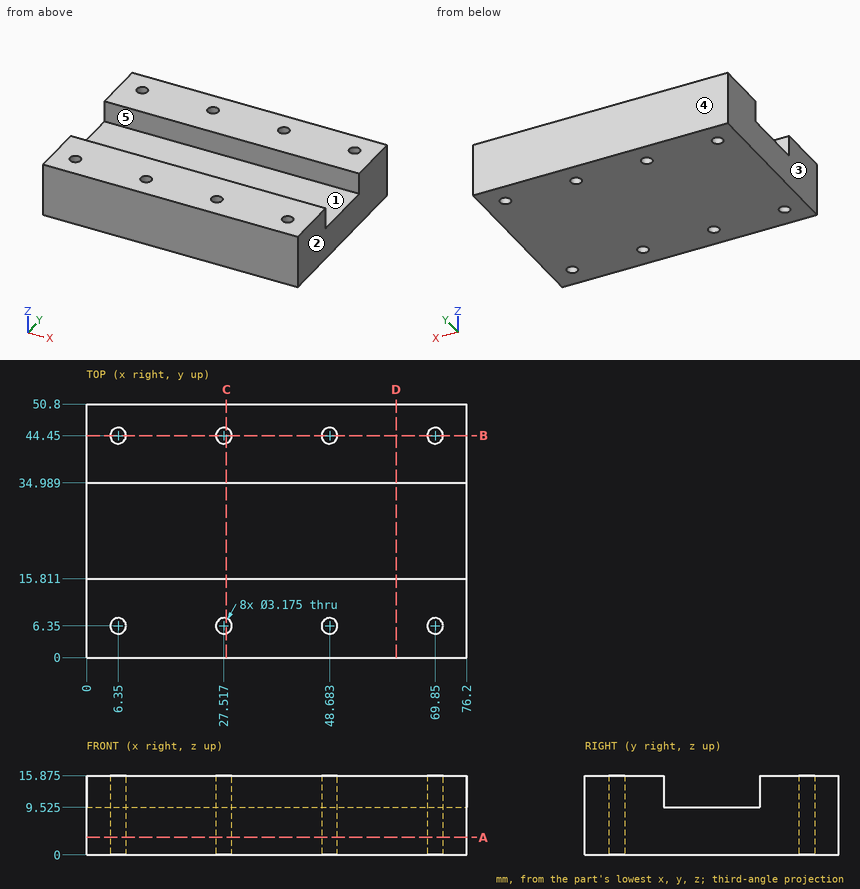
The drawing under review shows one solid part. Ordinate dimensions are in mm from its lowest x, y, z. A direction names the side the tool comes from. Give positions to 0.01 mm unless a question says otherwise; leave off trailing zeros. Write each loop counter-clockwise with the first axis right and the second up, starting at its lowest first coordinate (ties: lowest second). Pieces come first, ordered by that corner, then holes.
1. Add section D-D, the plane x = 62. Write out the cut boundary in (y, z) (1 decimal).
2. Draft analysis for pull direction Y (two halves, no side actions). For the marked faces 3, 4 and 5, state which applies: +Y half, -Y half, draft (parallel to the pull), parting line (faces both ways), or undercut.
3. Tool access review of the marked faces 1 and 2: name each direction out of +Z, -Z, +X, -X, +Y, -Y from which nothing blocks a thin tool from reaching the whole face with its end or side.
4. Add section C-C, the plane x = 28. Write out the cut boundary in (y, z) (1 decimal).
5. Wall thickness on L1, parallel to Y at x = 69.85, z = 10; L2, parallel to X at y = 44.45, z = 6 (1 decimal); L3, parallel to Y at x = 6.35, z = 6: over which ranges is each line inside the solid? List them lowest first.
6. Add section A-A, the plane z = 3.5. Count the separate pieces of the cut face and the enclosed holes in it, plus the area to 3 significant figures.
7. Add section B-B, the plane y = 44.45. Write out the cut boundary in (x, z) (1 decimal).
Worked answers:
1. outline: (0, 0) - (50.8, 0) - (50.8, 15.9) - (35, 15.9) - (35, 9.5) - (15.8, 9.5) - (15.8, 15.9) - (0, 15.9) - close
2. face 3: draft
2. face 4: +Y half
2. face 5: undercut
3. face 1: +Z, +X, -X
3. face 2: +Z, -Z, +X, +Y, -Y
4. outline: (0, 0) - (4.8, 0) - (4.8, 15.9) - (0, 15.9) - close; (7.9, 0) - (42.9, 0) - (42.9, 15.9) - (35, 15.9) - (35, 9.5) - (15.8, 9.5) - (15.8, 15.9) - (7.9, 15.9) - close; (46, 0) - (50.8, 0) - (50.8, 15.9) - (46, 15.9) - close
5. L1: y = 0 to 4.76, 7.94 to 15.81, 34.99 to 42.86, 46.04 to 50.8
5. L2: x = 0 to 4.8, 7.9 to 25.9, 29.1 to 47.1, 50.3 to 68.3, 71.4 to 76.2
5. L3: y = 0 to 4.76, 7.94 to 42.86, 46.04 to 50.8
6. separate pieces: 1
6. enclosed holes: 8
6. area: 3,810 mm2
7. outline: (0, 0) - (4.8, 0) - (4.8, 15.9) - (0, 15.9) - close; (7.9, 0) - (25.9, 0) - (25.9, 15.9) - (7.9, 15.9) - close; (29.1, 0) - (47.1, 0) - (47.1, 15.9) - (29.1, 15.9) - close; (50.3, 0) - (68.3, 0) - (68.3, 15.9) - (50.3, 15.9) - close; (71.4, 0) - (76.2, 0) - (76.2, 15.9) - (71.4, 15.9) - close
